The model under review builds one solid part; all positions refer to its coordinate system, in mm. A direction names the side the tool comes from. Round coordinates to 2 decimals unless told otherwise and drop trailing zeros. Loops run counter-clockwise (first coordinate to the right, second up) from the corner with the lowest first, then second, coordinate; pieces in that order, holes last. Notation, with made-up numbers: (-21.5, 9) -> (12.5, 9) arc R30 cw to (12.5, 40) -> close; hole circle Ø5 at (57, 65.5). An arc over 180 degrees is marked (long way). Return JSON: item names as keys, results as strings. Group by question number.
Autodesk Inventor part; units mm, degrees
ref_plane "Work Plane1" through (-51.0014, -51.0767, 47.0039) normal (0, 0, -1) x (0, 1, 0)
ref_plane "YZ Plane" through (0, 0, 0) normal (1, 0, 0) x (0, 1, 0)
ref_plane "XZ Plane" through (0, 0, 0) normal (0, 1, 0) x (-1, 0, 0)
ref_plane "Work Plane1" through (-51.0014, -51.0767, 47.0039) normal (0, 0, -1) x (0, 1, 0)
sketch "Sketch1" plane through (0, 0, 0) normal (0, 0, 1) x (1, 0, 0)
  arc A0 (-51.0008, -8.0945) -> (-16.665, 27.298) centre (-36.8015, 12.4817) ccw
  line L0 (15.6539, 51.0767) -> (-36.8027, 12.4817)
  line L1 (-36.8027, 12.4817) -> (-51.0008, 12.4817)
  line L2 (-51.0008, 12.4817) -> (-51.0008, -51.0767)
  line L3 (-15.3897, 25.4817) -> (-29.0068, 25.4817)
  line L4 (-14.1984, 25.4817) -> (-15.3897, 25.4817)
  ellipse E0 centre (-22.3234, 16.4817) end of major axis (-22.3234, 28.6067) minor radius 12.125 (-14.1984, 7.4817) -> (-14.1984, 25.4817) ccw
  line L5 (-15.3897, 7.4817) -> (-14.1984, 7.4817)
  line L6 (-29.0068, 7.4817) -> (-15.3897, 7.4817)
  line L7 (-30.1984, 7.4817) -> (-29.0068, 7.4817)
  ellipse E1 centre (-22.0734, 16.4817) end of major axis (-22.0734, 4.3567) minor radius 12.125 (-30.1984, 25.4817) -> (-30.1984, 7.4817) ccw
  line L8 (-44.552, -10.5183) -> (-37.9322, -10.5183)
  line L9 (-37.9322, -10.5183) -> (-35.1718, -10.5183)
  line L10 (-35.1718, -10.5183) -> (-28.552, -10.5183)
  arc A1 (-28.552, -10.5183) -> (-24.6451, -3.0183) centre (-36.677, -1.5183) ccw
  arc A2 (-28.552, -10.5183) -> (-28.552, 7.4817) centre (-36.677, -1.5183) ccw
  line L11 (-35.2148, 7.4817) -> (-28.552, 7.4817)
  line L12 (-35.2148, 7.4817) -> (-37.8892, 7.4817)
  line L13 (-44.552, 7.4817) -> (-37.8892, 7.4817)
  arc A3 (-44.552, 7.4817) -> (-46.3273, 5.4817) centre (-36.427, -1.5183) ccw
  ellipse E2 centre (-36.4279, -1.5183) end of major axis (-36.4279, -13.1433) minor radius 11.625 (-44.3583, 6.9817) -> (-44.3583, -10.0183) ccw
  arc A4 (-46.3273, 5.4817) -> (-48.4589, -0.0183) centre (-36.427, -1.5183) ccw
  arc A5 (-44.552, 7.4817) -> (-44.552, -10.5183) centre (-36.427, -1.5183) ccw
  point P0 (0, 0)
  point P1 (-11.8976, 10.2915)
  point P2 (-34.0379, 14.5159)
  point P3 (-15.4473, 25.4817)
  point P4 (-19.1337, 25.4817)
  point P5 (-16.6653, 27.2981)
  point P6 (-51.0008, -8.0945)
  dimension "d0" = 50
extrude "Extrusion1" add sketch "Sketch1" along normal up to surface (47.0015 mm away) contours L2 L1 L0 E1 L11 L12 L13 A3 A4 A5 L8 L9 L10 A1 A2 L6 L5 E0 A0
properties part number "ROTATE"
1. We need section C-C, the plane x = -15. Write out the cut boundary in (y, z).
2. We need section B-B, the plane x = -36. Write out the cut boundary in (y, z), then the cut area to 3 significant figures.
3. Wall thickness on line 1 (X direction, y = 1, z = 34); line 2 (X direction, y = 0.5, z = 10.5); line 3 (Y direction, x = -47, z = 45.5): over which ranges is each line inside the solid? List them lowest first.
4. For P1, Ø11.5, axis at x = -43, z = 19, coming from the +Y side; P2, Ø8, axis at x = -24.5, z = 8, coming from the -Y side; P3, Ø5, axis at x = -16.5, z = 35.5, coming from the -Y side, all flat-tipped, find the tip position at first contact; note any pin that passes through.
5. We need section D-D, the plane x = -20.5. Write out the cut boundary in (y, z), then the cut area to 3 significant figures.
6. Draft analysis for pull direction Y (two halves, no side actions). For faces 1 (the face through (-21, 7.482, 23)), 2 (the face through (-51.001, 2, 23)), 3 (the face through (-25.896, -7.066, 23.172)), state which applies: pulls with the +Y half, pulls with the -Y half, needs draft (parallel to the pull), parting line crosses it, or undercut.
7. We need section A-A, the plane y = -2.25. Write out the cut boundary in (x, z).
8. Tool access review of faces 4 (the face through (-44, 12.482, 23)), 5 (the face through (-34, 8, 0)), 6 (the face through (-45.507, 6.517, 23.172)): name each direction out of +Z, -Z, +X, -X, +Y, -Y from which nothing blocks a thin tool from reaching the whole face with its end or side.
Check sheet entries:
{
 "1": {"outline": "(0.25, 0) -> (7.48, 0) -> (7.48, 47) -> (0.25, 47) -> close"},
 "2": {"outline": "(-12.51, 0) -> (-10.52, 0) -> (-10.52, 47) -> (-12.51, 47) -> close; (7.48, 0) -> (13.07, 0) -> (13.07, 47) -> (7.48, 47) -> close", "area": "356 mm²"},
 "3": {"line 1": "x = -51 to -48.29, -24.82 to -14.59", "line 2": "x = -51 to -48.38, -24.72 to -14.86", "line 3": "y = -10.34 to -7.45, 4.42 to 12.48"},
 "4": {"P1": "stops at y = 12.48", "P2": "stops at y = -11.1", "P3": "stops at y = -5.07"},
 "5": {"outline": "(-6.47, 0) -> (7.48, 0) -> (7.48, 47) -> (-6.47, 47) -> close", "area": "656 mm²"},
 "6": {"face 1": "pulls with the +Y half", "face 2": "needs draft", "face 3": "undercut"},
 "7": {"outline": "(-51, 0) -> (-48.53, 0) -> (-48.53, 47) -> (-51, 47) -> close; (-24.57, 0) -> (-16.6, 0) -> (-16.6, 47) -> (-24.57, 47) -> close"},
 "8": {"face 4": "+Z, -Z, -X, +Y", "face 5": "-Z, +X, -X, +Y, -Y", "face 6": "+Z, -Z"}
}
